```python
from build123d import *

# Parameters (mm, degrees)
BOSS_EXTRUDE1_DEPTH = 50.8
CUT_EXTRUDE1_REACH  = 89.586


with BuildPart() as part:
    # Sketch1 → Boss-Extrude1 (new body)
    with BuildSketch(Plane.XY):
        Polygon((52.45808334, -3.175), (52.45808334, -60.325), (46.10808334, -60.325), (46.10808334, -9.525), (20.70808334, -9.525), (20.70808334, -60.325), (14.35808334, -60.325), (14.35808334, -3.175), align=None)
    extrude(amount=-BOSS_EXTRUDE1_DEPTH)

    # Cut-Extrude1: up to this face of the body (flat: up to its plane)
    cut_extrude1_end = Plane(part.part.faces().sort_by_distance((52.45808334, -31.75, -25.4))[0])
    # Sketch2 → Cut-Extrude1 (cut, up to the picked face)
    with BuildSketch(Plane.ZY.offset(-14.35808334), mode=Mode.PRIVATE) as cut_extrude1_sk1:
        with BuildLine():
            ThreePointArc((-22.225, -53.975), (-23.15493597, -51.72993597), (-25.4, -50.8))
            Line((-25.4, -50.8), (-25.4, -57.15))
            ThreePointArc((-25.4, -57.15), (-23.15493597, -56.22006403), (-22.225, -53.975))
        make_face()
    cut_extrude1_tool1 = split(extrude(cut_extrude1_sk1.sketch, amount=-CUT_EXTRUDE1_REACH, mode=Mode.PRIVATE), bisect_by=cut_extrude1_end, keep=Keep.BOTH, mode=Mode.PRIVATE)
    # Sketch2 → Cut-Extrude1 (cut, up to the picked face)
    with BuildSketch(Plane.ZY.offset(-14.35808334), mode=Mode.PRIVATE) as cut_extrude1_sk2:
        with BuildLine():
            Line((-25.4, -57.15), (-25.4, -50.8))
            ThreePointArc((-25.4, -50.8), (-28.575, -53.975), (-25.4, -57.15))
        make_face()
    cut_extrude1_tool2 = split(extrude(cut_extrude1_sk2.sketch, amount=-CUT_EXTRUDE1_REACH, mode=Mode.PRIVATE), bisect_by=cut_extrude1_end, keep=Keep.BOTH, mode=Mode.PRIVATE)
    # Sketch2 → Cut-Extrude1 (cut, up to the picked face)
    with BuildSketch(Plane.ZY.offset(-14.35808334), mode=Mode.PRIVATE) as cut_extrude1_sk3:
        with BuildLine():
            ThreePointArc((-22.225, -53.975), (-23.15493597, -51.72993597), (-25.4, -50.8))
            Line((-25.4, -50.8), (-25.4, -57.15))
            ThreePointArc((-25.4, -57.15), (-23.15493597, -56.22006403), (-22.225, -53.975))
        make_face()
    cut_extrude1_tool3 = split(extrude(cut_extrude1_sk3.sketch, amount=-CUT_EXTRUDE1_REACH, mode=Mode.PRIVATE), bisect_by=cut_extrude1_end, keep=Keep.BOTH, mode=Mode.PRIVATE)
    # Sketch2 → Cut-Extrude1 (cut, up to the picked face)
    with BuildSketch(Plane.ZY.offset(-14.35808334), mode=Mode.PRIVATE) as cut_extrude1_sk4:
        with BuildLine():
            Line((-25.4, -57.15), (-25.4, -50.8))
            ThreePointArc((-25.4, -50.8), (-28.575, -53.975), (-25.4, -57.15))
        make_face()
    cut_extrude1_tool4 = split(extrude(cut_extrude1_sk4.sketch, amount=-CUT_EXTRUDE1_REACH, mode=Mode.PRIVATE), bisect_by=cut_extrude1_end, keep=Keep.BOTH, mode=Mode.PRIVATE)
    # Sketch2 → Cut-Extrude1 (cut, up to the picked face)
    with BuildSketch(Plane.ZY.offset(-14.35808334), mode=Mode.PRIVATE) as cut_extrude1_sk5:
        with BuildLine():
            Line((0, -9.643805147), (-19.540665388, -56.422590224))
            ThreePointArc((-19.540665388, -56.422590224), (-21.880035364, -59.260106334), (-25.4, -60.325))
            Line((-25.4, -60.325), (0, -60.325))
            Line((0, -60.325), (0, -9.643805147))
        make_face()
    cut_extrude1_tool5 = split(extrude(cut_extrude1_sk5.sketch, amount=-CUT_EXTRUDE1_REACH, mode=Mode.PRIVATE), bisect_by=cut_extrude1_end, keep=Keep.BOTH, mode=Mode.PRIVATE)
    # Sketch2 → Cut-Extrude1 (cut, up to the picked face)
    with BuildSketch(Plane.ZY.offset(-14.35808334), mode=Mode.PRIVATE) as cut_extrude1_sk6:
        with BuildLine():
            ThreePointArc((-25.4, -60.325), (-28.919964636, -59.260106334), (-31.259334612, -56.422590224))
            Line((-31.259334612, -56.422590224), (-50.8, -9.643805147))
            Line((-50.8, -9.643805147), (-50.8, -60.325))
            Line((-50.8, -60.325), (-25.4, -60.325))
        make_face()
    cut_extrude1_tool6 = split(extrude(cut_extrude1_sk6.sketch, amount=-CUT_EXTRUDE1_REACH, mode=Mode.PRIVATE), bisect_by=cut_extrude1_end, keep=Keep.BOTH, mode=Mode.PRIVATE)
    add(cut_extrude1_tool1.solids().sort_by(Axis((14.358083, -53.975, -24.052488), (1, 0, 0)))[0], mode=Mode.SUBTRACT)
    add(cut_extrude1_tool2.solids().sort_by(Axis((14.358083, -53.975, -26.747512), (1, 0, 0)))[0], mode=Mode.SUBTRACT)
    add(cut_extrude1_tool3.solids().sort_by(Axis((14.358083, -53.975, -24.052488), (1, 0, 0)))[0], mode=Mode.SUBTRACT)
    add(cut_extrude1_tool4.solids().sort_by(Axis((14.358083, -53.975, -26.747512), (1, 0, 0)))[0], mode=Mode.SUBTRACT)
    add(cut_extrude1_tool5.solids().sort_by(Axis((14.358083, -43.525452, -7.142919), (1, 0, 0)))[0], mode=Mode.SUBTRACT)
    add(cut_extrude1_tool6.solids().sort_by(Axis((14.358083, -43.525452, -43.657081), (1, 0, 0)))[0], mode=Mode.SUBTRACT)


solid = part.part
```
Can you work these out from the model? Positions are in its coordinate system, mm. A direction names the side the tool comes from. Round coordinates to 2 decimals unless told otherwise and drop trailing zeros. Loops run counter-clockwise (first coordinate to the right, second up) from the corner with the lowest first, then second, coordinate; pieces in that order, holes last.
Item 1: If we mould it in two halves opening along X, with no side actions, what happens to faces 1 (the flat face through (14.358, -26, -25)), 2 (the flat face through (17.489, -33.361, -40.893)), 3 (the flat face through (20.708, -29, -25))? For each: +X half, -X half, draft (parallel to the pull), parting line (faces both ways), or undercut.
Item 2: Will these pins go through, and if not, where does the flat tip stop? pin 1 Ø8 at (x, z) = (41, -10) entering from -Y (3 decimals); pin 2 Ø4 at (x, y) = (45, -26) entering from +Z.
Item 3: Please list where these lines run through material, in increasing order: L1, parallel to X at y = -14, z = -7; L2, parallel to Y at x = 26.5, z = -17.5 (3 decimals); L3, parallel to Y at x = 51, z = -22.5 (3 decimals).
Item 4: Suppose I cut it at D-D, the plane z = -7. Write out the boundary of the cut face in (x, y) (3 decimals), then the cut area to 3 significant figures.
Item 5: Which directions (+Z, -Z, +X, -X, +Y, -Y) give clear straight access to the entire face, cutting with the end or side of a thin tool? Please do faces 4 (the flat face through (34, -6, 0)), 5 (the flat face through (46.108, -30, -25)).
Item 6: Suppose I cut it at C-C, the plane z = -27. Write out the boundary of the cut face in (x, y) (3 decimals).
Item 7: Suppose I cut it at B-B, the plane y = -50. Write out the boundary of the cut face in (x, z), then the cut area to 3 significant figures.
Item 8: Suppose I cut it at A-A, the plane x = 17.5. Write out the boundary of the cut face in (y, z) (3 decimals), then the cut area to 3 significant figures.
Reported:
1. face 1: -X half
1. face 2: draft
1. face 3: undercut
2. pin 1: stops at y = -9.525
2. pin 2: stops at z = -6.14
3. L1: x = 14.36 to 20.71, 46.11 to 52.46
3. L2: y = -9.525 to -3.175
3. L3: y = -59.624 to -55.268, -52.682 to -3.175
4. outline: (14.358, -26.401) - (20.708, -26.401) - (20.708, -9.525) - (46.108, -9.525) - (46.108, -26.401) - (52.458, -26.401) - (52.458, -3.175) - (14.358, -3.175) - close
4. area: 456 mm2
5. face 4: +Z, +X, -X, +Y, -Y
5. face 5: +Z, -Z, -Y
6. outline: (14.358, -60.12) - (20.708, -60.12) - (20.708, -56.717) - (14.358, -56.717) - close; (14.358, -51.233) - (20.708, -51.233) - (20.708, -9.525) - (46.108, -9.525) - (46.108, -51.233) - (52.458, -51.233) - (52.458, -3.175) - (14.358, -3.175) - close; (46.108, -60.12) - (52.458, -60.12) - (52.458, -56.717) - (46.108, -56.717) - close
7. outline: (14.36, -33.94) - (20.71, -33.94) - (20.71, -16.86) - (14.36, -16.86) - close; (46.11, -33.94) - (52.46, -33.94) - (52.46, -16.86) - (46.11, -16.86) - close
7. area: 217 mm2
8. outline: (-56.423, -31.259) - (-9.644, -50.8) - (-3.175, -50.8) - (-3.175, 0) - (-9.644, 0) - (-56.423, -19.541) arc R6.35 ccw to start; hole circle Ø6.35 at (-53.975, -25.4)
8. area: 1,790 mm2
